The model under review builds one solid part; all positions refer to its coordinate system, in mm. Face numbers are marked on the shaded views. Coordinates: 2 decimals unless noted, no trailing zeros. Write each loop counter-clockwise with the first axis right and the second up, starting at its lowest first coordinate (ties: lowest second). Pieces come first, ordered by that corner, then holes. Notation, with made-up numbers: (7.5, -30) -> (65.5, -30) arc R16 ccw to (65.5, -6) -> close; hole circle Ø7 at (86.25, -7.75). An arc over 180 degrees is marked (long way). Write each question's results on one line, items separated by ' | '.
```python
from build123d import *

# Parameters (mm, degrees)
SKETCH1_R           = 119.5
BOSS_EXTRUDE1_DEPTH = 7
CHAMFER2_SIZE       = 10
SKETCH3_R           = 108
CUT_EXTRUDE1_DEPTH  = 2
SKETCH4_R           = 90
SKETCH4_R_2         = 2
CUT_EXTRUDE2_DEPTH  = 165.904517828


with BuildPart() as part:
    # Sketch1 → Boss-Extrude1 (new body)
    with BuildSketch(Plane.XY):
        Circle(SKETCH1_R)
    extrude(amount=BOSS_EXTRUDE1_DEPTH)

    # Chamfer2
    # the kernel refuses this chamfer: 10 mm, written as the material it takes off along each edge
    with BuildSketch(Plane(origin=(0, 0, 7), x_dir=(1, 0, 0), z_dir=(0, -1, 0))) as chamfer2_piece_1:
        Polygon((119.5, -CHAMFER2_SIZE), (119.5 - CHAMFER2_SIZE, 0), (119.5, 0), align=None)
    revolve(axis=Axis((0, 0, 7), (0, 0, 1)), mode=Mode.SUBTRACT)

    # Sketch3 → Cut-Extrude1 (cut)
    with BuildSketch(Plane.XY.offset(7)):
        Circle(SKETCH3_R)
    extrude(amount=-CUT_EXTRUDE1_DEPTH, mode=Mode.SUBTRACT)

    # Sketch4 → Cut-Extrude2 (cut, through all)
    with BuildSketch(Plane(origin=(0, 0, 0), x_dir=(-1, 0, 0), z_dir=(0, 0, -1))):
        Circle(SKETCH4_R)
        with Locations((0, 98)):
            Circle(SKETCH4_R_2)
        with Locations((84.870489571, 49)):
            Circle(SKETCH4_R_2)
        with Locations((84.870489571, -49)):
            Circle(SKETCH4_R_2)
        with Locations((0, -98)):
            Circle(SKETCH4_R_2)
        with Locations((-84.870489571, -49)):
            Circle(SKETCH4_R_2)
        with Locations((-84.870489571, 49)):
            Circle(SKETCH4_R_2)
    extrude(amount=-CUT_EXTRUDE2_DEPTH, mode=Mode.SUBTRACT)


solid = part.part
```
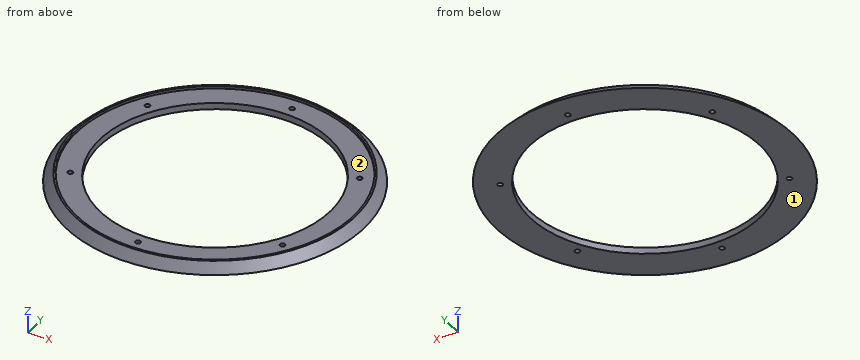
Q1. Clearance check with flat-ended pins moving along their axes: P1, Ø3, axis at x = -84.87, y = 49, coming from the -Z side; P2, Ø1, axis at x = 69.5, z = 4, coming from the +Y side; P3, Ø6.5, axis at x = 84.87, y = -49, coming from the +Z side; P4, Ø3, axis at y = 37.5, z = 3.5, coming from the +X side. State where each tip first meets the part, or that it passes through.
Solution:
P1: through | P2: y = 89.21 | P3: z = 5 | P4: x = 108.27
Q2. Draft analysis for pull direction Y (two halves, no side actions). For the marked faces 1 and 2, state which applies: pulls with the +Y half, pulls with the -Y half, needs draft (parallel to the pull), parting line crosses it, or undercut.
Solution:
face 1: needs draft | face 2: undercut
Q3. For line 1 (X direction, y = -51.5, z = 4.25); line 2 (X direction, y = -69.5, z = 6.25); line 3 (Y direction, x = 13, z = 2.5), list the stretches that pass through material, from the lowest coordinate up. Write a range as from..to.
Solution:
line 1: -99.74..-73.81, 73.81..99.74 | line 2: -85.59..-82.67, 82.67..85.59 | line 3: -113.26..-89.06, 89.06..113.26
Q4. Add section A-A (y = 0). Write out the cut boundary in (x, z), plus the area to 3 significant figures.
Solution:
outline: (-116.5, 0) -> (-90, 0) -> (-90, 5) -> (-108, 5) -> (-108, 7) -> (-109.5, 7) -> close; (90, 0) -> (116.5, 0) -> (109.5, 7) -> (108, 7) -> (108, 5) -> (90, 5) -> close | area: 250 mm²
